Here's the drawing with two shaded views (mm, measured from the low corner). I have some questions. A direction names the side the tool comes from. Coordinates: 2 decimals unless noted, no trailing zeros. Write each loop counter-clockwise with the first axis right and the second up, starting at its lowest first coordinate (ties: lowest second). Pieces come first, ordered by that corner, then holes.
Item 1: I'm going to push flat-ended pins straight in: pin 1 Ø5 at (y, z) = (11, 25) entering from +X; pin 2 Ø8 at (y, z) = (19.5, 6) entering from -X. Where does each tip first touch, or does it pass through?
Item 2: If we section it at A-A (z = 22.5): Please give me the cut outline in (x, y), then the cut area to 3 significant figures.
Item 3: We'd pull the mould along X, two halves only. Please class the marked faces 1 and 2: +X half, -X half, draft (parallel to the pull), parting line (faces both ways), or undercut.
Item 4: If we section it at D-D (z = 8): Please give me the cut outline in (x, y), then the cut area to 3 significant figures.
Item 5: If we section it at C-C (x = 250): Please give me the cut outline in (y, z).
Item 6: If we section it at B-B (y = 8): Please give me the cut outline in (x, z), then the cut area to 3 significant figures.
Item 7: For the marked faces 3, 4 and 5, which set-ups out of +Z, -Z, +X, -X, +Y, -Y let a thin tool reach every point of the face, with its end or its side?
Item 8: If I drill on line 1 (X direction, y = 3.5, z = 23); line 2 (X direction, y = 15, z = 23.5); line 3 (Y direction, x = 20.5, z = 5.5), over which ranges is the centre line in solid material (lowest first)?
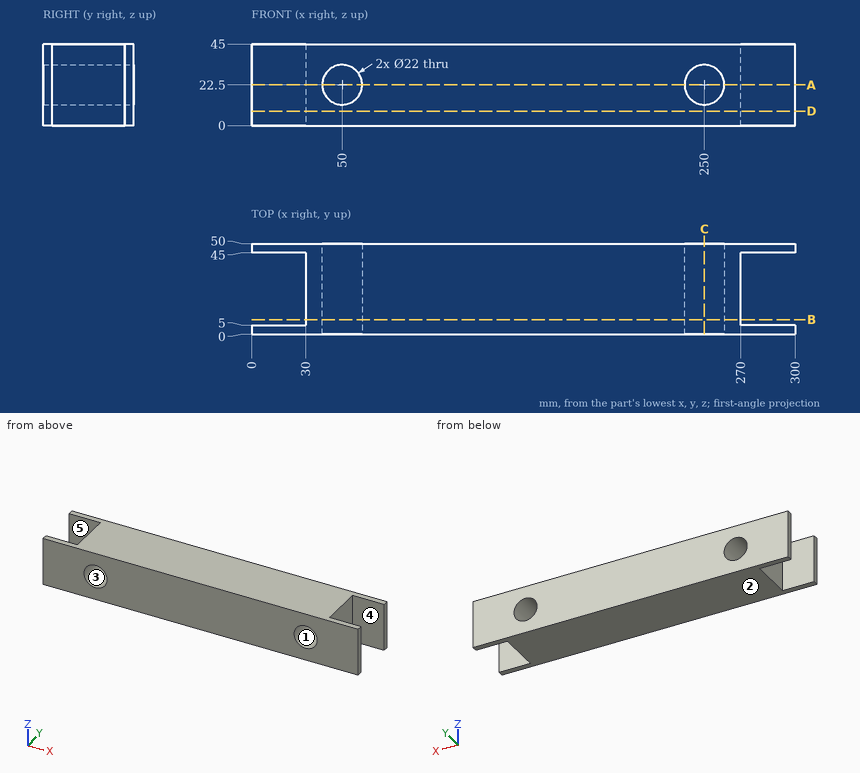
Answer list:
1. pin 1: stops at x = 270
1. pin 2: stops at x = 30
2. outline: (0, 0) - (39, 0) - (39, 50) - (0, 50) - (0, 45) - (30, 45) - (30, 5) - (0, 5) - close; (61, 0) - (239, 0) - (239, 50) - (61, 50) - close; (261, 0) - (300, 0) - (300, 5) - (270, 5) - (270, 45) - (300, 45) - (300, 50) - (261, 50) - close
2. area: 10,400 mm2
3. face 1: undercut
3. face 2: draft
4. outline: (0, 0) - (300, 0) - (300, 5) - (270, 5) - (270, 45) - (300, 45) - (300, 50) - (0, 50) - (0, 45) - (30, 45) - (30, 5) - (0, 5) - close
4. area: 12,600 mm2
5. outline: (0, 0) - (50, 0) - (50, 11.5) - (0, 11.5) - close; (0, 33.5) - (50, 33.5) - (50, 45) - (0, 45) - close
6. outline: (30, 0) - (270, 0) - (270, 45) - (30, 45) - close; hole circle Ø22 at (50, 22.5); hole circle Ø22 at (250, 22.5)
6. area: 10,000 mm2
7. face 3: +Y, -Y
7. face 4: +Z, -Z, +X
7. face 5: +Z, -Z, -X
8. line 1: x = 0 to 39.01, 60.99 to 239.01, 260.99 to 300
8. line 2: x = 30 to 39.05, 60.95 to 239.05, 260.95 to 270
8. line 3: y = 0 to 5, 45 to 50
